Geometry: see drawing. Coordinates: mm, zero at the bounding-box minimum. A direction names the side the tool comes from. Coordinates: 2 decimals unless noted, no trailing zeros. Order: outer loops, then holes, each group sorted by start corner. A loop starts at its lowest first (then second) coordinate and runs counter-clockwise, first axis right, second up. Notation, with made-up numbers: M 83,0 L 129,0 A27 ccw 129,17 Z; hole C -6.75,20 d5. An arc over 180 degrees is marked long. Answer in a Markdown table with one row per item.
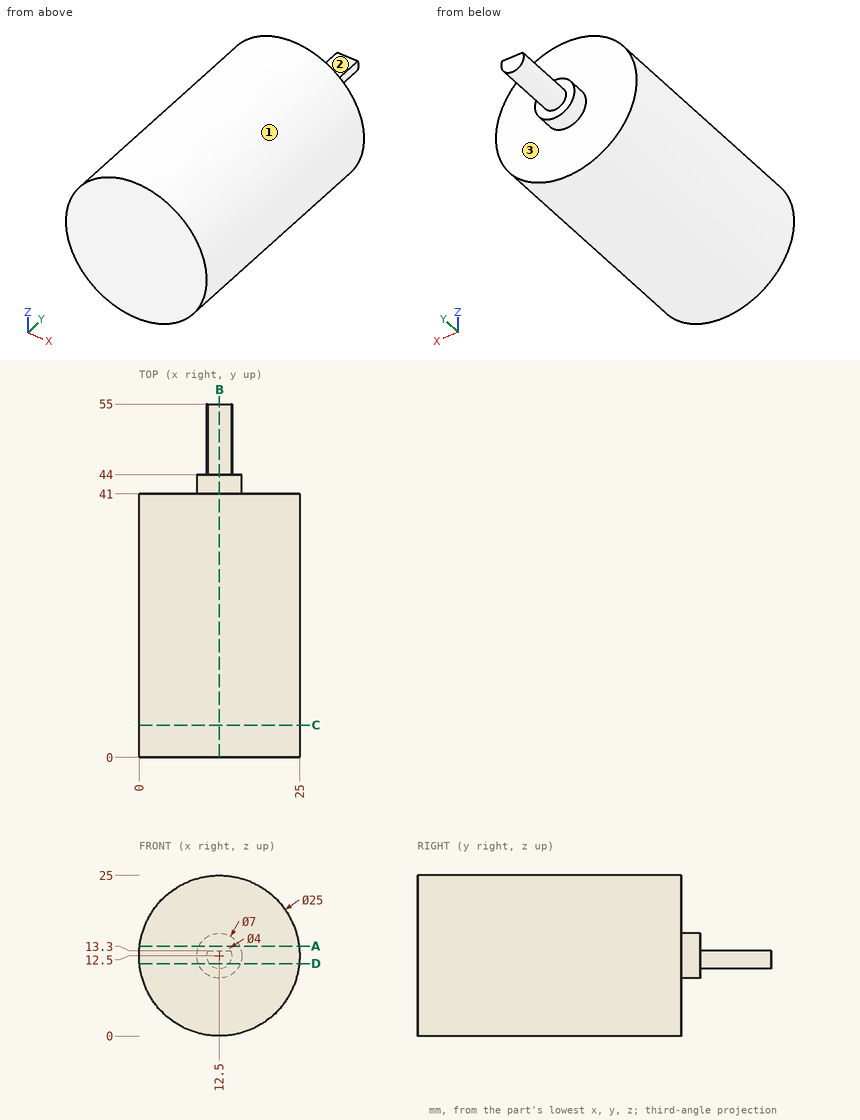
1) Reachability of the marked faces 1, 2 and 3 from +Z, -Z, +X, -X, +Y, -Y: full face, straight path, thin tool, end or side. Return the list, or none.
Resolved:
| item | result |
|---|---|
| face 1 | +Y, -Y |
| face 2 | +Z, +X, -X, +Y |
| face 3 | +Y |
2) Cut plane B-B, the plane x = 12.5. Output: boundary loops of the cut face in (y, z).
Resolved:
| item | result |
|---|---|
| outline | M 0,0 L 41,0 L 41,9 L 44,9 L 44,10.5 L 55,10.5 L 55,13.3 L 44,13.3 L 44,16 L 41,16 L 41,25 L 0,25 Z |
3) Material intervals for probe 1 along Y at (x, z) = (16, 11.25); probe 2 along X at (y, z) = (28, 12.75); probe 3 along Z at (x, y) = (22.75, 20), sorted ascending.
Resolved:
| item | result |
|---|---|
| probe 1 | y = 0 to 41 |
| probe 2 | x = 0 to 25 |
| probe 3 | z = 5.35 to 19.65 |
4) Cut plane D-D, the plane z = 11.25. Output: boundary loops of the cut face in (x, y), and give its area (3 significant figures).
Resolved:
| item | result |
|---|---|
| outline | M 0.06,0 L 24.94,0 L 24.94,41 L 15.77,41 L 15.77,44 L 14.06,44 L 14.06,55 L 10.94,55 L 10.94,44 L 9.23,44 L 9.23,41 L 0.06,41 Z |
| area | 1,070 mm2 |
5) Contact query for flat-ended pins moving along their axis: pin 1 (10 mm diameter, centred on y = 40.5, z = 2.5, fed in from -X); pin 2 (1 mm diameter, centred on x = 20.5, y = 28.5, fed in from +Z); pin 3 (12 mm diameter, centred on x = 5.5, z = 22, fed in from +Y); pin 4 (10 mm diameter, centred on x = 22, y = 47, fed in from -Z). Output: stop coordinate, or through.
Resolved:
| item | result |
|---|---|
| pin 1 | stops at x = 1.04 |
| pin 2 | stops at z = 22.5 |
| pin 3 | stops at y = 41 |
| pin 4 | passes through |
6) Cut plane C-C, the plane y = 5. Output: boundary loops of the cut face in (x, z).
Resolved:
| item | result |
|---|---|
| outline | C 12.5,12.5 d25 |
7) Cut plane A-A, the plane z = 14. Output: boundary loops of the cut face in (x, y).
Resolved:
| item | result |
|---|---|
| outline | M 0.09,0 L 24.91,0 L 24.91,41 L 15.66,41 L 15.66,44 L 9.34,44 L 9.34,41 L 0.09,41 Z |
